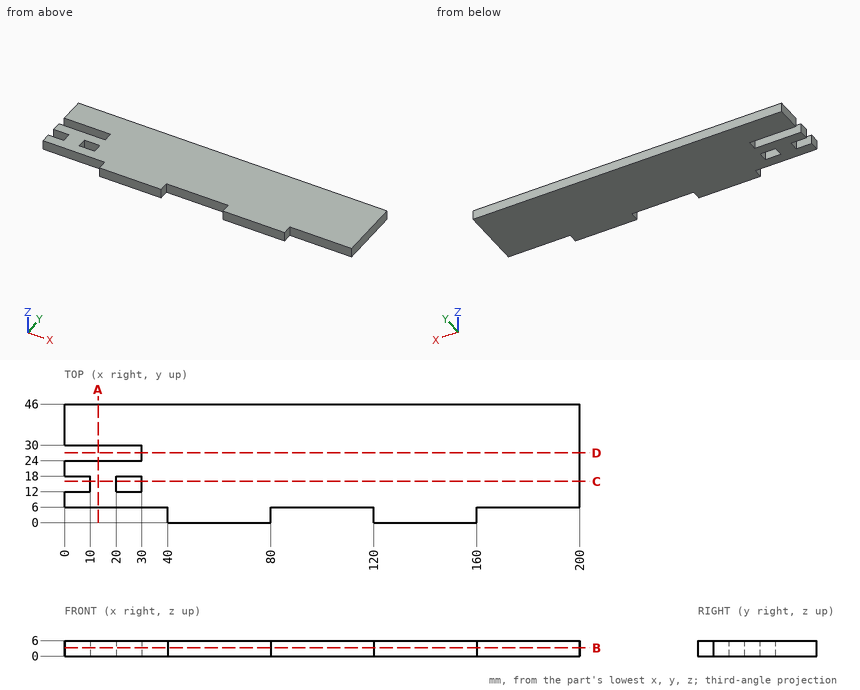
Input: dimensioned drawing with shaded views. Units: mm. Origin: part minimum x, y, z. Coordinates: 2 decimals unless noted, no trailing zeros. Order: outer loops, then holes, each group sorted by start corner. A loop starts at its lowest first (then second) coordinate and runs counter-clockwise, first axis right, second up. Notation, with made-up numbers: (82, 39) -> (105, 39) arc R31 cw to (105, 70) -> close; hole circle Ø3 at (20, 16). An arc over 180 degrees is marked (long way). Answer in a Markdown table with one row per item.
Item 1: Section B-B on z = 3.15. Output: boundary loops of the cut face in (x, y).
Return value:
| item | result |
|---|---|
| outline | (0, 6) -> (40, 6) -> (40, 0) -> (80, 0) -> (80, 6) -> (120, 6) -> (120, 0) -> (160, 0) -> (160, 6) -> (200, 6) -> (200, 46) -> (0, 46) -> (0, 30) -> (30, 30) -> (30, 24) -> (0, 24) -> (0, 18) -> (10, 18) -> (10, 12) -> (0, 12) -> close; hole (20, 12) -> (30, 12) -> (30, 18) -> (20, 18) -> close |
Item 2: Section D-D on y = 27. Output: boundary loops of the cut face in (x, z), plus the area to 3 significant figures.
Return value:
| item | result |
|---|---|
| outline | (30, 0) -> (200, 0) -> (200, 6) -> (30, 6) -> close |
| area | 1,020 mm² |
Item 3: Section C-C on y = 16. Output: boundary loops of the cut face in (x, z), plus the area to 3 significant figures.
Return value:
| item | result |
|---|---|
| outline | (10, 0) -> (20, 0) -> (20, 6) -> (10, 6) -> close; (30, 0) -> (200, 0) -> (200, 6) -> (30, 6) -> close |
| area | 1,080 mm² |
Item 4: Ray query, L1, parallel to X at y = 17.5, z = 3.5; L2, parallel to Y at x = 13, z = 3.85; L3, parallel to X at y = 2.5, z = 5.15. Return the intervals inside material, ascending.
Return value:
| item | result |
|---|---|
| L1 | x = 10 to 20, 30 to 200 |
| L2 | y = 6 to 24, 30 to 46 |
| L3 | x = 40 to 80, 120 to 160 |
Item 5: Section A-A on x = 13. Output: boundary loops of the cut face in (y, z), plus the area to 3 significant figures.
Return value:
| item | result |
|---|---|
| outline | (6, 0) -> (24, 0) -> (24, 6) -> (6, 6) -> close; (30, 0) -> (46, 0) -> (46, 6) -> (30, 6) -> close |
| area | 204 mm² |
Item 6: Contact query for flat-ended pins moving along their axis: P1, Ø3, axis at x = 29, z = 2.5, coming from the -Y side; P2, Ø1.8, axis at y = 3.5, z = 4, coming from the +X side; P3, Ø1.8, axis at y = 2, z = 3.5, coming from the -X side. Output: stop coordinate, or through.
Return value:
| item | result |
|---|---|
| P1 | stops at y = 6 |
| P2 | stops at x = 160 |
| P3 | stops at x = 40 |
